```python
from build123d import *

# Parameters (mm, degrees)
SKETCH1_W           = 3.5
SKETCH1_H           = 4
SKETCH2_R           = 2
BOSS_EXTRUDE1_DEPTH = 16
CUT_EXTRUDE1_DEPTH  = 2.4


with BuildPart() as part:
    # Sketch1 → Revolve1 (revolve)
    with BuildSketch(Plane.XZ, mode=Mode.PRIVATE) as revolve1_sk:
        with Locations((1.75, 2)):
            Rectangle(SKETCH1_W, SKETCH1_H)
    revolve(revolve1_sk.sketch.rotate(Axis((0, 0, 4), (0, 0, -1)), 180), axis=Axis((0, 0, 4), (0, 0, -1)))

    # Sketch2 → Boss-Extrude1 (add)
    with BuildSketch(Plane.XY.offset(4)):
        Circle(SKETCH2_R)
    extrude(amount=BOSS_EXTRUDE1_DEPTH)

    # Sketch3 → Cut-Extrude1 (cut)
    with BuildSketch(Plane(origin=(0, 0, 0), x_dir=(-1, 0, 0), z_dir=(0, 0, -1))):
        Polygon((-1.7, 0), (-0.85, -1.472243186), (0.85, -1.472243186), (1.7, 0), (0.85, 1.472243186), (-0.85, 1.472243186), align=None)
    extrude(amount=-CUT_EXTRUDE1_DEPTH, mode=Mode.SUBTRACT)


solid = part.part
```
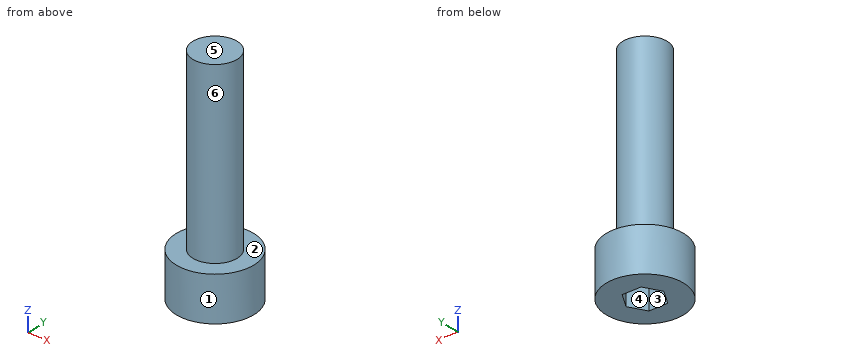
CAD build for the part. Positions are in the model's coordinates, mm. Face numbers are marked on the shaded views. A direction names the side the tool comes from. Coordinates: 2 decimals unless noted, no trailing zeros. Write each loop counter-clockwise with the first axis right and the second up, starting at its lowest first coordinate (ties: lowest second). Pieces come first, ordered by that corner, then holes. Notation, with made-up numbers: (-9.5, 29) -> (17.5, 29) arc R16 cw to (17.5, 52) -> close; hole circle Ø7 at (59.5, 89). An arc over 180 degrees is marked (long way). Return JSON: item names as keys, results as strings. Group by question number.
Q1. Which spindle directions (+Z, -Z, +X, -X, +Y, -Y) get a long thin tool onto all of the face, cutting with end or side? Do the marked faces 4, 5 and 6. Say none if no direction does.
Q2. Drill centre lines: line 1 (Y direction, x = 1, z = 1); line 2 (Z direction, x = 0.5, y = -2.5); line 3 (Z direction, x = 1, y = 0.5). Where is each one in solid material? Low to high.
Q3. Cut at B-B, the plane y = 1.75. Give the cut face in (x, z).
Q4. Flat gauge pins, fed straight in: pin 1 (3 mm diameter, centred on x = -2.5, y = 2.5, fed in from +Z); pin 2 (3 mm diameter, centred on x = 0.5, y = 0, fed in from -Z); pin 3 (0.5 mm diameter, centred on x = 0.5, z = 1.5, fed in from -Y). Where does each tip first touch, or does it go through?
Q5. Cut at C-C, the plane z = 9.5. Give the cut face in (x, y), then the cut area to 3 significant figures.
Q6. Cut at A-A, the plane x = 0. Give the cut face in (y, z), then the cut area to 3 significant figures.
Q7. Pull direction X, two halves, no side cores. Call the marked faces 1, 2 and 3: released by +X, released by -X, zero draft, split by the parting line, or undercut.
Q8. Cut at D-D, the plane x = 1.25. Give the cut face in (y, z).
Returned:
{
 "1": {"face 4": "-Z", "face 5": "+Z, +X, -X, +Y, -Y", "face 6": "+Z"},
 "2": {"line 1": "y = -3.35 to -1.21, 1.21 to 3.35", "line 2": "z = 0 to 4", "line 3": "z = 2.4 to 20"},
 "3": {"outline": "(-3.03, 0) -> (3.03, 0) -> (3.03, 4) -> (0.97, 4) -> (0.97, 20) -> (-0.97, 20) -> (-0.97, 4) -> (-3.03, 4) -> close"},
 "4": {"pin 1": "stops at z = 4", "pin 2": "stops at z = 0", "pin 3": "stops at y = -3.49"},
 "5": {"outline": "circle Ø4 at (0, 0)", "area": "12.6 mm2"},
 "6": {"outline": "(-3.5, 0) -> (-1.47, 0) -> (-1.47, 2.4) -> (1.47, 2.4) -> (1.47, 0) -> (3.5, 0) -> (3.5, 4) -> (2, 4) -> (2, 20) -> (-2, 20) -> (-2, 4) -> (-3.5, 4) -> close", "area": "84.9 mm2"},
 "7": {"face 1": "split by the parting line", "face 2": "zero draft", "face 3": "undercut"},
 "8": {"outline": "(-3.27, 0) -> (-0.78, 0) -> (-0.78, 2.4) -> (0.78, 2.4) -> (0.78, 0) -> (3.27, 0) -> (3.27, 4) -> (1.56, 4) -> (1.56, 20) -> (-1.56, 20) -> (-1.56, 4) -> (-3.27, 4) -> close"}
}
